```python
from build123d import *

# Parameters (mm, degrees)
CYLINDER034_R           = 5.5
CYLINDER034_DEPTH       = 10
CYLINDER034_PITCH_ANGLE = 90
CYLINDER_R              = 6
CYLINDER_DEPTH          = 10
CYLINDER_PITCH_ANGLE    = 90


with BuildPart() as cylinder034:
    # Cylinder034 → Cylinder034 (new body)
    with BuildSketch(Plane.XY):
        Circle(CYLINDER034_R)
    extrude(amount=CYLINDER034_DEPTH)


with BuildPart() as cylinder034_1:
    # Cylinder034 pitch: moved
    add(cylinder034.part.rotate(Axis((0, 0, 0), (0, 1, 0)), CYLINDER034_PITCH_ANGLE))


with BuildPart() as cylinder034_2:
    # Cylinder034 placement: moved
    add(cylinder034_1.part.moved(Location((3, 84, 11.5))))


with BuildPart() as cut059:
    # Cylinder → Cylinder (new body)
    with BuildSketch(Plane.XY):
        Circle(CYLINDER_R)
    extrude(amount=CYLINDER_DEPTH)


with BuildPart() as cut059_1:
    # Cylinder pitch: moved
    add(cut059.part.rotate(Axis((0, 0, 0), (0, 1, 0)), CYLINDER_PITCH_ANGLE))


with BuildPart() as cut059_2:
    # Cylinder placement: moved
    add(cut059_1.part.moved(Location((3, 84, 11.5))))

    # Cut059: cut Cylinder034
    add(cylinder034_2.part, mode=Mode.SUBTRACT)


solid = cut059_2.part
```
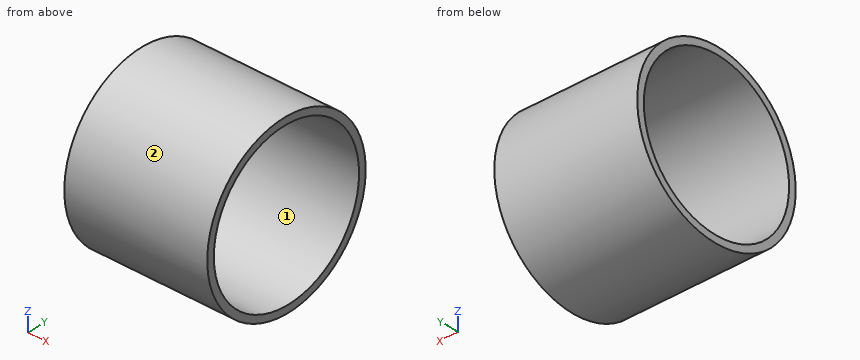
Model file for the job. Use its own axes, mm. Face numbers are marked on the shaded views. Give positions to 0.01 mm unless a question says otherwise; leave off trailing zeros. Write each loop counter-clockwise with the first axis right and the second up, starting at its lowest first coordinate (ties: lowest second). Pieces come first, ordered by that corner, then holes. Notation, with made-up numbers: M 32.25,68 L 82.25,68 A22 ccw 82.25,106 Z; hole C -28.5,33 d4. An arc over 180 degrees is marked long. Use a Markdown table: item, result.
1) Cut at B-B (z = 11.5). List the corners of the cut face in (x, y).
Responses:
| item | result |
|---|---|
| outline | M 3,78 L 13,78 L 13,78.5 L 3,78.5 Z; M 3,89.5 L 13,89.5 L 13,90 L 3,90 Z |
2) Cut at C-C (x = 11.5). List the corners of the cut face in (y, z), and give its area (3 significant figures).
Responses:
| item | result |
|---|---|
| outline | C 84,11.5 d12; hole C 84,11.5 d11 |
| area | 18.1 mm2 |
3) Drill centre lines: line 1 (Y direction, x = 12.25, z = 11.5); line 2 (Y direction, x = 6.5, z = 8); line 3 (Z direction, x = 8.25, y = 79.5). Where is each one in solid material? Low to high. Write a range as from..to.
Responses:
| item | result |
|---|---|
| line 1 | y = 78..78.5, 89.5..90 |
| line 2 | y = 79.13..79.76, 88.24..88.87 |
| line 3 | z = 7.53..8.34, 14.66..15.47 |
4) Pin check, flat tips, straight feed: pin 1 (3 mm diameter, centred on x = 8, z = 7.5, fed in from +Y); pin 2 (1.5 mm diameter, centred on x = 8.5, z = 12.5, fed in from +Y); pin 3 (1.5 mm diameter, centred on y = 80, z = 14.5, fed in from +X). Stop position of each tip, or through.
Responses:
| item | result |
|---|---|
| pin 1 | stops at y = 89.45 |
| pin 2 | stops at y = 89.99 |
| pin 3 | stops at x = 13 |
5) Pull direction Z, two halves, no side cores. Call the marked faces 1 and 2: +Z half, -Z half, draft (parallel to the pull), parting line (faces both ways), or undercut.
Responses:
| item | result |
|---|---|
| face 1 | undercut |
| face 2 | parting line |
6) Cut at A-A (y = 84). List the corners of the cut face in (x, z).
Responses:
| item | result |
|---|---|
| outline | M 3,5.5 L 13,5.5 L 13,6 L 3,6 Z; M 3,17 L 13,17 L 13,17.5 L 3,17.5 Z |
